Check sheet for the modelled part. Datum: model origin and axes. Units: mm. Give positions to 0.01 mm unless a question says otherwise; leave off trailing zeros. Order: outer loops, then holes, each group sorted by start corner. A loop starts at its lowest first (then second) coordinate and runs counter-clockwise, first axis right, second up. Notation, with made-up numbers: (40.5, -8) -> (72.5, -8) arc R17 ccw to (72.5, 6) -> close; hole circle Ø6 at (-15, 46). An arc over 180 degrees is marked (long way). Answer in a Markdown table with one row per item. Add a question column.
(1) Cross-section at C-C (z = 5.25). State how many separate pieces and enclosed holes the cut face has, then the cut area to 3 significant figures.
(2) Cross-section at B-B (y = 367.5). Record the cut outline in (x, z), then the cut area to 3 significant figures.
(3) Cross-section at A-A (x = 172). Record the cut outline in (y, z).
(4) Thickness scan on L1, parallel to Y at x = 185, z = 6.25; L2, parallel to Y at x = 51.5, z = 7.5; L3, parallel to X at y = 594, z = 6.5 (3 decimals). Record the ranges inside material, lowest first. Write a range as [from, to].
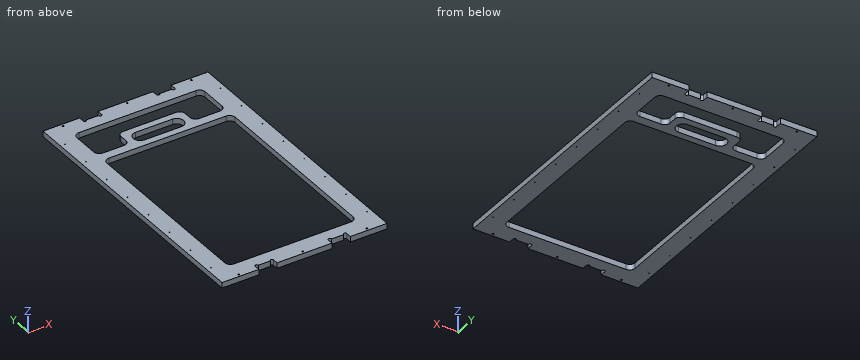
```python
from build123d import *

# Parameters (mm, degrees)
F0_R     = 1.75
F0_R_2   = 1
F1_DEPTH = 12


with BuildPart() as f1:
    # F0 (on Top) → F1 (new body)
    with BuildSketch(Plane.XY):
        with BuildLine():
            Line((0, 600), (0, 0))
            Line((0, 0), (80, 0))
            Line((80, 0), (80, 12))
            ThreePointArc((80, 12), (83.5, 15.5), (87, 12))
            Line((87, 12), (113, 12))
            ThreePointArc((113, 12), (116.5, 15.5), (120, 12))
            Line((120, 12), (120, 0))
            Line((120, 0), (239.85, 0))
            Line((239.85, 0), (239.85, 12))
            ThreePointArc((239.85, 12), (243.35, 15.5), (246.85, 12))
            Line((246.85, 12), (272.85, 12))
            ThreePointArc((272.85, 12), (276.35, 15.5), (279.85, 12))
            Line((279.85, 12), (279.85, 0))
            Line((279.85, 0), (359.85, 0))
            Line((359.85, 0), (359.85, 600))
            Line((359.85, 600), (279.85, 600))
            Line((279.85, 600), (279.85, 588))
            ThreePointArc((279.85, 588), (276.35, 584.5), (272.85, 588))
            Line((272.85, 588), (246.85, 588))
            ThreePointArc((246.85, 588), (243.35, 584.5), (239.85, 588))
            Line((239.85, 588), (239.85, 600))
            Line((239.85, 600), (120, 600))
            Line((120, 600), (120, 588))
            ThreePointArc((120, 588), (116.5, 584.5), (113, 588))
            Line((113, 588), (87, 588))
            ThreePointArc((87, 588), (83.5, 584.5), (80, 588))
            Line((80, 588), (80, 600))
            Line((80, 600), (0, 600))
        make_face()
        with Locations((40, 6)):
            Circle(F0_R, mode=Mode.SUBTRACT)
        with Locations((10, 52)):
            Circle(F0_R_2, mode=Mode.SUBTRACT)
        with Locations((10, 122)):
            Circle(F0_R_2, mode=Mode.SUBTRACT)
        with Locations((10, 192)):
            Circle(F0_R_2, mode=Mode.SUBTRACT)
        with Locations((10, 262)):
            Circle(F0_R_2, mode=Mode.SUBTRACT)
        with Locations((179.925, 6)):
            Circle(F0_R, mode=Mode.SUBTRACT)
        with Locations((319.85, 6)):
            Circle(F0_R, mode=Mode.SUBTRACT)
        with Locations((349.85, 52)):
            Circle(F0_R_2, mode=Mode.SUBTRACT)
        with Locations((349.85, 122)):
            Circle(F0_R_2, mode=Mode.SUBTRACT)
        with BuildLine():
            ThreePointArc((40, 447.265898), (43.514719, 455.75118), (52, 459.265898))
            Line((52, 459.265898), (307.85, 459.265898))
            ThreePointArc((307.85, 459.265898), (316.335281, 455.75118), (319.85, 447.265898))
            Line((319.85, 447.265898), (319.85, 52))
            ThreePointArc((319.85, 52), (316.335281, 43.514719), (307.85, 40))
            Line((307.85, 40), (52, 40))
            ThreePointArc((52, 40), (43.514719, 43.514719), (40, 52))
            Line((40, 52), (40, 447.265898))
        make_face(mode=Mode.SUBTRACT)
        with Locations((349.85, 192)):
            Circle(F0_R_2, mode=Mode.SUBTRACT)
        with Locations((349.85, 262)):
            Circle(F0_R_2, mode=Mode.SUBTRACT)
        with Locations((10, 332)):
            Circle(F0_R_2, mode=Mode.SUBTRACT)
        with Locations((10, 402)):
            Circle(F0_R_2, mode=Mode.SUBTRACT)
        with Locations((10, 472)):
            Circle(F0_R_2, mode=Mode.SUBTRACT)
        with Locations((10, 542)):
            Circle(F0_R_2, mode=Mode.SUBTRACT)
        with Locations((40, 594)):
            Circle(F0_R, mode=Mode.SUBTRACT)
        with Locations((349.85, 332)):
            Circle(F0_R_2, mode=Mode.SUBTRACT)
        with Locations((349.85, 402)):
            Circle(F0_R_2, mode=Mode.SUBTRACT)
        with BuildLine():
            Line((219.85, 474.265898), (140, 474.265898))
            ThreePointArc((140, 474.265898), (125, 489.265898), (140, 504.265898))
            Line((140, 504.265898), (219.85, 504.265898))
            ThreePointArc((219.85, 504.265898), (234.85, 489.265898), (219.85, 474.265898))
        make_face(mode=Mode.SUBTRACT)
        with BuildLine():
            ThreePointArc((40, 548), (43.514719, 556.485281), (52, 560))
            Line((52, 560), (307.85, 560))
            ThreePointArc((307.85, 560), (316.335281, 556.485281), (319.85, 548))
            Line((319.85, 548), (319.85, 491.265898))
            ThreePointArc((319.85, 491.265898), (316.335281, 482.780617), (307.85, 479.265898))
            Line((307.85, 479.265898), (261.85, 479.265898))
            ThreePointArc((261.85, 479.265898), (253.364719, 482.780617), (249.85, 491.265898))
            Line((249.85, 491.265898), (249.85, 507.265898))
            ThreePointArc((249.85, 507.265898), (246.335281, 515.75118), (237.85, 519.265898))
            Line((237.85, 519.265898), (122, 519.265898))
            ThreePointArc((122, 519.265898), (113.514719, 515.75118), (110, 507.265898))
            Line((110, 507.265898), (110, 491.265898))
            ThreePointArc((110, 491.265898), (106.485281, 482.780617), (98, 479.265898))
            Line((98, 479.265898), (52, 479.265898))
            ThreePointArc((52, 479.265898), (43.514719, 482.780617), (40, 491.265898))
            Line((40, 491.265898), (40, 548))
        make_face(mode=Mode.SUBTRACT)
        with Locations((179.925, 594)):
            Circle(F0_R, mode=Mode.SUBTRACT)
        with Locations((349.85, 472)):
            Circle(F0_R_2, mode=Mode.SUBTRACT)
        with Locations((349.85, 542)):
            Circle(F0_R_2, mode=Mode.SUBTRACT)
        with Locations((319.85, 594)):
            Circle(F0_R, mode=Mode.SUBTRACT)
    extrude(amount=F1_DEPTH)


solid = f1.part
```
Answer below:
| question | item | result |
|---|---|---|
| 1 | separate pieces | 1 |
| 1 | enclosed holes | 25 |
| 1 | area | 76,500 mm² |
| 2 | outline | (0, 0) -> (40, 0) -> (40, 12) -> (0, 12) -> close; (319.85, 0) -> (359.85, 0) -> (359.85, 12) -> (319.85, 12) -> close |
| 2 | area | 960 mm² |
| 3 | outline | (0, 0) -> (40, 0) -> (40, 12) -> (0, 12) -> close; (459.27, 0) -> (474.27, 0) -> (474.27, 12) -> (459.27, 12) -> close; (504.27, 0) -> (519.27, 0) -> (519.27, 12) -> (504.27, 12) -> close; (560, 0) -> (600, 0) -> (600, 12) -> (560, 12) -> close |
| 4 | L1 | y = [0, 40], [459.27, 474.27], [504.27, 519.27], [560, 600] |
| 4 | L2 | y = [0, 40.01], [459.26, 479.28], [559.99, 600] |
| 4 | L3 | x = [0, 38.25], [41.75, 80], [120, 178.175], [181.675, 239.85], [279.85, 318.1], [321.6, 359.85] |
